from build123d import *

# Parameters (mm, degrees)
SKETCH_1_W          = 50
SKETCH_1_H          = 25
EXTRUDE_1_DEPTH     = 11
CUT_EXTRUDE_1_DEPTH = 53.699620492
CUT_EXTRUDE_2_DEPTH = 53.699620492
SKETCH_6_R          = 8
EXTRUDE_4_DEPTH     = 2.5
SKETCH_9_R          = 3
SKETCH_9_R_2        = 1.1
CUT_EXTRUDE_4_DEPTH = 2.5
SKETCH_12_R         = 2.2
CUT_EXTRUDE_5_DEPTH = 2
SKETCH_11_R         = 2.2
CUT_EXTRUDE_6_DEPTH = 2
SKETCH_13_R         = 8.2
CUT_EXTRUDE_7_DEPTH = 2.5
SKETCH_14_R         = 3
SKETCH_14_R_2       = 1.1
CUT_EXTRUDE_8_DEPTH = 2.5
CUT_EXTRUDE_9_DEPTH = 25
FILLET_1_R          = 1.2


with BuildPart() as part:
    # 草图1 → 凸台-拉伸1 (new body)
    with BuildSketch(Plane(origin=(0, 0, 0), x_dir=(1, 0, 0), z_dir=(0, 1, 0))):
        Rectangle(SKETCH_1_W, SKETCH_1_H)
    extrude(amount=EXTRUDE_1_DEPTH)

    # 草图2 → 切除-拉伸1 (cut, through all)
    with BuildSketch(Plane(origin=(25, 0, 0), x_dir=(0, 0, -1), z_dir=(1, 0, 0))):
        with BuildLine():
            Line((-12.5, 0), (-6.5, 0))
            ThreePointArc((-6.5, 0), (-10.742640687, 1.757359313), (-12.5, 6))
            Line((-12.5, 6), (-12.5, 0))
        make_face()
        with BuildLine():
            Line((12.5, 6), (12.5, 0))
            Line((12.5, 0), (6.5, 0))
            ThreePointArc((6.5, 0), (10.742640687, 1.757359313), (12.5, 6))
        make_face()
    extrude(amount=-CUT_EXTRUDE_1_DEPTH, mode=Mode.SUBTRACT)

    # 草图3 → 切除-拉伸2 (cut, through all)
    with BuildSketch(Plane(origin=(25, 0, 0), x_dir=(0, 0, -1), z_dir=(1, 0, 0))):
        with BuildLine():
            Line((-10, 11), (10, 11))
            Line((10, 11), (10, 2.429285786))
            ThreePointArc((10, 2.429285786), (8.390294809, 1.371092404), (6.5, 1))
            Line((6.5, 1), (-6.5, 1))
            ThreePointArc((-6.5, 1), (-8.390294809, 1.371092404), (-10, 2.429285786))
            Line((-10, 2.429285786), (-10, 11))
        make_face()
    extrude(amount=-CUT_EXTRUDE_2_DEPTH, mode=Mode.SUBTRACT)

    # 草图6 → 凸台-拉伸4 (add)
    with BuildSketch(Plane(origin=(0, 0, -12.5), x_dir=(-1, 0, 0), z_dir=(0, 0, -1))):
        with Locations((25, 8)):
            Circle(SKETCH_6_R)
        with Locations((-25, 8)):
            Circle(SKETCH_6_R)
    extrude(amount=-EXTRUDE_4_DEPTH)

    # 草图9 → 切除-拉伸4 (cut)
    with BuildSketch(Plane.XY.offset(12.5)):
        with Locations((25, 8)):
            Circle(SKETCH_9_R)
        with Locations((10, 8)):
            Circle(SKETCH_9_R_2)
    extrude(amount=-CUT_EXTRUDE_4_DEPTH, mode=Mode.SUBTRACT)

    # 草图12 → 切除-拉伸5 (cut)
    with BuildSketch(Plane.XY.offset(12.5)):
        with Locations((10, 8)):
            Circle(SKETCH_12_R)
    extrude(amount=-CUT_EXTRUDE_5_DEPTH, mode=Mode.SUBTRACT)

    # 草图11 → 切除-拉伸6 (cut)
    with BuildSketch(Plane(origin=(0, 0, -12.5), x_dir=(-1, 0, 0), z_dir=(0, 0, -1))):
        with Locations((10, 8)):
            Circle(SKETCH_11_R)
    extrude(amount=-CUT_EXTRUDE_6_DEPTH, mode=Mode.SUBTRACT)

    # 草图13 → 切除-拉伸7 (cut)
    with BuildSketch(Plane.XY.offset(12.5)):
        with Locations((-25, 8)):
            Circle(SKETCH_13_R)
        with Locations((25, 8)):
            Circle(SKETCH_13_R)
    extrude(amount=-CUT_EXTRUDE_7_DEPTH, mode=Mode.SUBTRACT)

    # 草图14 → 切除-拉伸8 (cut)
    with BuildSketch(Plane(origin=(0, 0, -12.5), x_dir=(-1, 0, 0), z_dir=(0, 0, -1))):
        with Locations((25, 8)):
            Circle(SKETCH_14_R)
        with Locations((-25, 8)):
            Circle(SKETCH_14_R)
        with Locations((10, 8)):
            Circle(SKETCH_14_R_2)
    extrude(amount=-CUT_EXTRUDE_8_DEPTH, mode=Mode.SUBTRACT)

    # 草图15 → 切除-拉伸9 (cut)
    with BuildSketch(Plane.XY.offset(-10)):
        Polygon((25, 8), (25, 0), (17.002930857, -0.216529728), align=None)
        Polygon((-17.002930857, -0.216529728), (-25, 8), (-25, 0), align=None)
    extrude(amount=CUT_EXTRUDE_9_DEPTH, mode=Mode.SUBTRACT)

    # 圆角1
    fillet_1_edges = [part.edges().sort_by_distance(p)[0] for p in [
        (0, 11, 10),
        (0, 11, -10),
    ]]
    fillet(fillet_1_edges, radius=FILLET_1_R)


solid = part.part
Work out the finished part from the listing and answer in its coordinate system (mm). A direction names the side the tool comes from. Round coordinates to 2 decimals unless told otherwise and drop trailing zeros. Order: outer loops, then holes, each group sorted by start corner. A loop starts at its lowest first (then second) coordinate and runs counter-clockwise, first axis right, second up. Notation, with made-up numbers: M 57.5,-17.75 L 100.5,-17.75 A29 cw 100.5,15.25 Z; hole C 71,9 d3. An arc over 180 degrees is marked long. One line per item, written item: value.
Q1. For faces 5 (the face through (0.274, 1.381, -8.415)), 6 (the face through (17.854, 0.658, 0.392)), 7 (the face through (9, 9, 10.5)), determine the directions among +Z, -Z, +X, -X, +Y, -Y from which every point of the face is accessible in a straight line to the end or side of a thin tool.
Derived:
face 5: +X, -X, +Y
face 6: +Z, +X, -Y
face 7: +Z
Q2. Find section D-D on x = -1. Write down the section's boundary in (y, z), then the cut area to 3 significant figures.
Derived:
outline: M 0,-6.5 A6 ccw 6,-12.5 L 11,-12.5 L 11,-11.2 A1.2 ccw 9.8,-10 L 2.43,-10 A5 cw 1,-6.5 L 1,6.5 A5 cw 2.43,10 L 9.8,10 A1.2 ccw 11,11.2 L 11,12.5 L 6,12.5 A6 ccw 0,6.5 Z
area: 62.0 mm²
Q3. Find section A-A on x = -25. Write down the section's boundary in (y, z).
Derived:
outline: M 0,-12.5 L 5,-12.5 L 5,-10 L 0,-10 Z; M 11,-12.5 L 16,-12.5 L 16,-10 L 11,-10 Z
Q4. Straight lines are drawn through the part: line 1 (Z direction, x = -10, y = 6.5); line 2 (Z direction, x = 13, y = 9.75); line 3 (Z direction, x = 21, y = 2.25). For each, find the intervals that lie inside material, in ascending order.
Derived:
line 1: -10.5 to -10, 10 to 12.5
line 2: -12.5 to -10, 10 to 12.5
line 3: -12.5 to -10
Q5. Determine the mould class of faces 1 (the face through (-11.016, 7.579, -10.253)), 2 (the face through (0, 0, 0)), 3 (the face through (-0.243, 10.639, 10.342)), 4 (the face through (-9, 9, -10.5)) for opening direction Y: released by +Y, released by -Y, zero draft, split by the parting line, or undercut.
Derived:
face 1: undercut
face 2: released by -Y
face 3: released by +Y
face 4: undercut
Q6. Find section C-C on y = 4. Write down the section's boundary in (x, z), then the cut area to 3 significant figures.
Derived:
outline: M -31.93,-12.5 L -18.07,-12.5 L -18.07,-12.16 L 18.07,-12.16 L 18.07,-12.5 L 31.93,-12.5 L 31.93,-10 L -31.93,-10 Z; M -17.84,10 L 17.84,10 L 17.84,12.16 L -17.84,12.16 Z
area: 224 mm²
Q7. Find section B-B on y = 8. Give the number of separate pieces and of enclosed holes in the cut face, then the cut area to 3 significant figures.
Derived:
separate pieces: 6
enclosed holes: 0
area: 199 mm²
Q8. Flat-ended cylindrical pins translate along their axes: pin 1 (1.3 mm diameter, centred on x = -10, y = 8, fed in from -Z); pin 2 (10.5 mm diameter, centred on x = -2, z = 3, fed in from +Y); pin 3 (6 mm diameter, centred on x = -25, y = 7.5, fed in from -Z); pin 4 (12 mm diameter, centred on x = 17, z = 2, fed in from +Y). Find the tip coordinate at first contact, or state that the pin passes through.
Derived:
pin 1: z = 10
pin 2: y = 1.32
pin 3: z = -12.5
pin 4: y = 1.23
